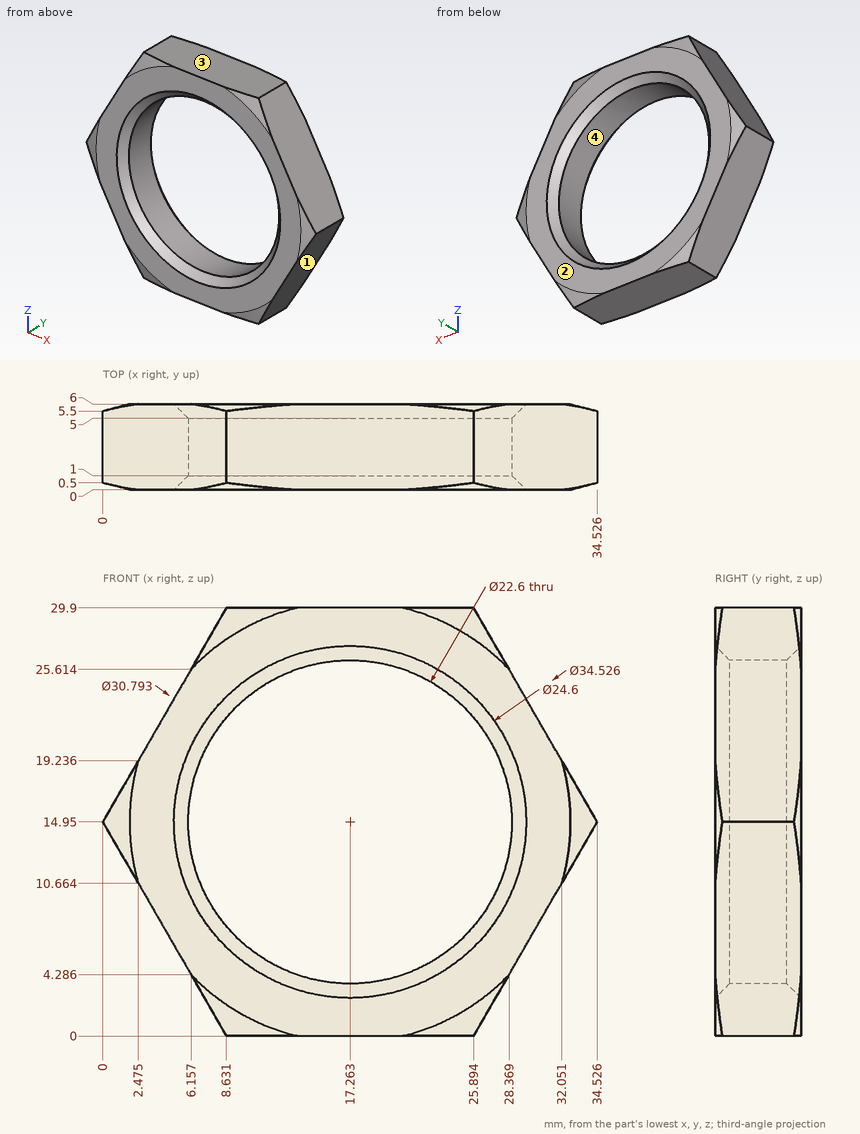
Geometry check sheet. Reference: drawing and pictorial views, mm from the part's lowest x, y, z. Round coordinates to 2 decimals unless told otherwise and drop trailing zeros.
1. Gauge pin test, flat ends, axial feed: P1, Ø10, axis at x = 15.5, z = 24, coming from the -Y side; P2, Ø3, axis at y = 1.5, z = 13, coming from the +X side (1 decimal). Record the tip position at first contact, or that the pin passes through.
2. Draft check along Z on the marked faces 1, 2, 3 and 4. Enter one of: +Z half, -Z half, draft (parallel to the pull), parting line (faces both ways), or undercut.
3. Scan lines: L1, parallel to Z at x = 22.5, y = 3.25 (1 decimal); L2, parallel to Z at x = 7.5, y = 2.5; L3, parallel to X at y = 3.5, z = 9.5 (1 decimal). Record each from-to range of solid material in increasing order.
Answer:
1. P1: stops at y = 0
1. P2: stops at x = 34.3
2. face 1: -Z half
2. face 2: draft
2. face 3: +Z half
2. face 4: undercut
3. L1: z = 0 to 4.9, 25 to 29.9
3. L2: z = 1.96 to 9.26, 20.64 to 27.94
3. L3: x = 3.1 to 7.4, 27.2 to 31.4
